from build123d import *

# Parameters (mm, degrees)
SKETCH1_W           = 5.334
SKETCH1_H           = 12.7
BOSS_EXTRUDE1_DEPTH = 5.334


with BuildPart() as part:
    # Sketch1 → Boss-Extrude1 (new body)
    with BuildSketch(Plane.XY):
        with BuildLine():
            Line((-9.525, 0), (-25.4, 0))
            ThreePointArc((-25.4, 0), (0, -25.4), (25.4, 0))
            Line((25.4, 0), (9.525, 0))
            Line((9.525, 0), (9.525, 72.39))
            Line((9.525, 72.39), (-9.525, 72.39))
            Line((-9.525, 72.39), (-9.525, 0))
        make_face()
        with Locations((0, 53.34)):
            Rectangle(SKETCH1_W, SKETCH1_H, mode=Mode.SUBTRACT)
    extrude(amount=BOSS_EXTRUDE1_DEPTH)


solid = part.part
Geometry: final body of the model. Coordinates: model frame, mm. A direction names the side the tool comes from. Coordinates: 2 decimals unless noted, no trailing zeros. Order: outer loops, then holes, each group sorted by start corner. A loop starts at its lowest first (then second) coordinate and runs counter-clockwise, first axis right, second up.
1) Set-up query: faces 1 (the flat face through (2.667, 53, 3)), 2 (the cylindrical face through (-0.559, -25.394, 2.63)), 3 (the flat face through (-17, 0, 3)), 4 (the flat face through (9.525, 36, 3)), 5 (the flat face through (0, 72.39, 3)). Return all of +Z, -Z, +X, -X, +Y, -Y with unobstructed straight access to the full face (end or side cutting, diameter ignored); none if empty.
Result sheet:
face 1: +Z, -Z
face 2: +Z, -Z, -Y
face 3: +Z, -Z, -X, +Y
face 4: +Z, -Z, +X, +Y
face 5: +Z, -Z, +X, -X, +Y
2) Section A-A (y = 50.5). Return loops of the section in (x, z) (3 decimals).
Result sheet:
outline: (-9.525, 0) - (-2.667, 0) - (-2.667, 5.334) - (-9.525, 5.334) - close; (2.667, 0) - (9.525, 0) - (9.525, 5.334) - (2.667, 5.334) - close
3) Section B-B (x = 0). Return loops of the section in (y, z).
Result sheet:
outline: (-25.4, 0) - (46.99, 0) - (46.99, 5.33) - (-25.4, 5.33) - close; (59.69, 0) - (72.39, 0) - (72.39, 5.33) - (59.69, 5.33) - close
4) Ray query, probe 1 along X at (y, z) = (56, 1.55) (3 decimals); probe 2 along X at (y, z) = (15.5, 4.85) (3 decimals); probe 3 along Y at (x, z) = (15, 0.9). Return the intervals inside material, ascending.
Result sheet:
probe 1: x = -9.525 to -2.667, 2.667 to 9.525
probe 2: x = -9.525 to 9.525
probe 3: y = -20.5 to 0
5) Draft query along Y for faces 6 (the flat face through (0, 59.69, 3)), 7 (the flat face through (-2.667, 53, 3)), 8 (the flat face through (0, 13, 0)), 9 (the flat face through (18, 0, 3)). Return one class per face: released by +Y, released by -Y, zero draft, split by the parting line, or undercut.
Result sheet:
face 6: undercut
face 7: undercut
face 8: zero draft
face 9: released by +Y
6) Section D-D (y = -11). Return loops of the section in (x, z), then the cut area to 3 significant figures.
Result sheet:
outline: (-22.89, 0) - (22.89, 0) - (22.89, 5.33) - (-22.89, 5.33) - close
area: 244 mm2
7) First-contact query: P1, Ø1.5, axis at y = 45, z = 1, coming from the -X side (3 decimals); P2, Ø1.6, axis at x = -0.5, z = 1.5, coming from the -Y side; P3, Ø3, axis at x = 12, z = 2.5, coming from the -Y side. Flat tips, straight axial feed; report the tip coordinate or a pass-through.
Result sheet:
P1: stops at x = -9.525
P2: stops at y = -25.4
P3: stops at y = -23.13
8) Section C-C (z = 3.2). Return loops of the section in (x, y) (3 decimals), then the cut area to 3 significant figures.
Result sheet:
outline: (-25.4, 0) arc R25.4 ccw to (25.4, 0) - (9.525, 0) - (9.525, 72.39) - (-9.525, 72.39) - (-9.525, 0) - close; hole (-2.667, 46.99) - (2.667, 46.99) - (2.667, 59.69) - (-2.667, 59.69) - close
area: 2,320 mm2
